Geometry: final body of the model. Coordinates: model frame, mm. A direction names the side the tool comes from. Give positions to 0.01 mm unless a question says otherwise; leave off trailing zeros. Write each loop counter-clockwise with the first axis right and the second up, starting at its lowest first coordinate (ties: lowest second). Pieces come first, ordered by that corner, then holes. Notation, with made-up numbers: M 62,38.5 L 109,38.5 A19 ccw 109,59.5 Z; hole C 32,85 d2. An arc over 180 degrees is marked long. Use a Markdown table: item, result. Add a question column.
(1) Reachability of faces 3 (the flat face through (2, -5, -32)), 4 (the flat face through (15.304, 32.045, -19.867)), 5 (the flat face through (-20, 32, -32.483)), 6 (the flat face through (-16, 1, -12.797)) from +Z, -Z, +X, -X, +Y, -Y: full face, straight path, thin tool, end or side. Return the list, or none.
(2) Cut plane B-B (x = 0). Output: boundary loops of the cut face in (y, z).
(3) Pin query (flat end, axial travel): pin 1 Ø1.2 at (x, y) = (-16, 2) entering from +Z; pin 2 Ø1.2 at (x, z) = (-16.5, -17.5) entering from -Y; pin 3 Ø2.5 at (x, y) = (-16, 1) entering from -Z; pin 4 Ø22.5 at (x, z) = (1, -36.5) entering from -Y. Return the tip coordinate at first contact, or that it passes through.
(4) Cut plane D-D (y = 27.5). Output: boundary loops of the cut face in (x, z), plus the area to 3 significant figures.
(5) Cut plane A-A (z = 0). Output: boundary loops of the cut face in (x, y).
(6) Cut plane C-C (y = 18). Output: boundary loops of the cut face in (x, z).
(7) Material intervals for L1, parallel to Z at x = 0, y = -4; L2, parallel to Y at x = -7.5, z = 0; L3, parallel to Y at x = -19.5, z = -21, sorted ascending.
(8) Draft query along Z for faces 1 (the cylindrical face through (7.63, -3.52, -37.56)), 2 (the flat face through (-5, 65, -20)). Return one class per face: released by +Z, released by -Z, zero draft, split by the parting line, or undercut.
Autodesk Inventor part; units mm, degrees
ref_plane "YZ Plane" through (0, 0, 0) normal (1, 0, 0) x (0, 1, 0)
ref_plane "XZ Plane" through (0, 0, 0) normal (0, 1, 0) x (-1, 0, 0)
ref_plane "XY Plane" through (0, 0, 0) normal (0, 0, 1) x (1, 0, 0)
sketch "Esquisse7" plane through (0, 0, 0) normal (0, 1, 0) x (-1, 0, 0)
  circle A0 centre (0, 0) radius 15
  circle A1 centre (0, -39.9666) radius 15
  line L0 (13, -7.4833) -> (-13, -7.4833)
  line L1 (-13, -7.4833) -> (-13, -32.4833)
  line L2 (-13, -32.4833) -> (13, -32.4833)
  line L3 (13, -32.4833) -> (13, -7.4833)
  dimension "d39" = 30
  dimension "d40" = 25
  dimension "d41" = 26
extrude "Extrusion7" add sketch "Esquisse7" along normal blind 65
sketch "Esquisse8" plane through (-13, 0, -32.4833) normal (-1, 0, 0) x (0, 0, 1)
  line L0 (0, 0) -> (25, 0) construction
  line L1 (25, 0) -> (25, 65) construction
  line L2 (0, 65) -> (25, 65) construction
  line L3 (0, 0) -> (0, 65) construction
  line L4 (25, 0) -> (0, 0)
  line L5 (0, 0) -> (0, 65)
  line L6 (0, 65) -> (25, 65)
  line L7 (25, 65) -> (25, 0)
  point P0 (32.4833, 0)
extrude "Extrusion8" add sketch "Esquisse8" along normal blind 12
sketch "Esquisse9" plane through (0, 0, 0) normal (0, -1, 0) x (1, 0, 0)
  arc A0 (-13, -32.4833) -> (13, -32.4833) centre (0, -39.9666) ccw construction
  line L0 (13, -7.4833) -> (13, -32.4833) construction
  arc A1 (13, -7.4833) -> (-13, -7.4833) centre (0, 0) ccw construction
  line L1 (-13, -7.4833) -> (-25, -7.4833) construction
  line L2 (-25, -32.4833) -> (-25, -7.4833) construction
  line L3 (-13, -32.4833) -> (-25, -32.4833) construction
  line L4 (-13, -7.4833) -> (-25, -7.4833) construction
  line L5 (-15, -7.4833) -> (-15, -32.4833) construction
  line L6 (-13, -32.4833) -> (-25, -32.4833) construction
  line L7 (-15, -12.7966) -> (-17.3067, -12.7966)
  line L8 (-17.3067, -12.7966) -> (-17.3067, -27.5847)
  line L9 (-17.3067, -27.5847) -> (-15, -27.5847)
  line L10 (-15, -27.5847) -> (-15, -12.7966)
  point P0 (-15, -29.9833)
  dimension "d47" = 10
extrude "Extrusion9" cut sketch "Esquisse9" against normal blind 3
sketch "Esquisse10" plane through (0, 0, 0) normal (0, -1, 0) x (1, 0, 0)
  arc A0 (-13, -32.4833) -> (13, -32.4833) centre (0, -39.9666) ccw construction
  line L0 (13, -7.4833) -> (13, -32.4833) construction
  arc A1 (13, -7.4833) -> (-13, -7.4833) centre (0, 0) ccw construction
  line L1 (-13, -7.4833) -> (-25, -7.4833) construction
  line L2 (-25, -32.4833) -> (-25, -7.4833) construction
  line L3 (-13, -32.4833) -> (-25, -32.4833) construction
  circle A2 centre (0, 0) radius 11.5
  circle A3 centre (0, -39.9666) radius 11.5
  arc A4 (-13, -32.4833) -> (13, -32.4833) centre (0, -39.9666) ccw
  dimension "d58" = 23
extrude "Extrusion10" add sketch "Esquisse10" along normal blind 5
sketch "Esquisse11" plane through (0, -5, 0) normal (0, -1, 0) x (1, 0, 0)
  circle A0 centre (0, -39.9666) radius 11.5 construction
  circle A1 centre (0, 0) radius 11.5 construction
  circle A2 centre (0, 0) radius 8
  circle A3 centre (0, -39.9666) radius 8
  dimension "d54" = 16
extrude "Extrusion11" cut sketch "Esquisse11" against normal blind 3
fillet "Congé6" radius 20 2 edges at (13, 32.5, -7.4833) (13, 32.5, -32.4833)
draft "Dépouille de face1" angle 4 pull direction (0, 1, 0) faces at (13, 21.6667, -17.2095) (13.057, 21.6667, -29.813) (13.2275, 21.6667, -8.6539) (-14.4854, 43.3333, -43.862) (-14.0102, 43.3333, -5.3586) fixed edges at (13, 65, -19.9833) (13.2878, 65, -31.6853) (13.2878, 65, -8.2813) (-1.3678, 65, -54.9041) (-1.3678, 65, 14.9375)
properties part number "head1"
Answer list:
| question | item | result |
|---|---|---|
| 1 | face 3 | +Z, -Z, +X, -X, -Y |
| 1 | face 4 | +X, +Y |
| 1 | face 5 | -X, +Y |
| 1 | face 6 | -Y |
| 2 | outline | M -5,-51.47 L 0,-51.47 L 0,-59.51 L 65,-54.97 L 65,15 L 0,19.55 L 0,11.5 L -5,11.5 L -5,8 L -2,8 L -2,-8 L -5,-8 L -5,-11.5 L 0,-11.5 L 0,-28.47 L -5,-28.47 L -5,-31.97 L -2,-31.97 L -2,-47.97 L -5,-47.97 Z |
| 3 | pin 1 | z = 11.81 |
| 3 | pin 2 | y = 3 |
| 3 | pin 3 | z = -52.69 |
| 3 | pin 4 | y = -5 |
| 4 | outline | M -25,-32.48 L -15.95,-32.48 A17.62 ccw long 16.62,-34.09 A17.38 cw 15.62,-28.3 L 15.62,-11.66 A17.38 cw 16.62,-5.87 A17.62 ccw long -15.95,-7.48 L -25,-7.48 Z |
| 4 | area | 2,500 mm² |
| 5 | outline | M -19.55,0 L -11.5,0 L -11.5,-5 L -8,-5 L -8,-2 L 8,-2 L 8,-5 L 11.5,-5 L 11.5,0 L 19.55,0 L 15,65 L -15,65 Z |
| 6 | outline | M -25,-32.48 L -16.69,-32.48 A18.29 ccw long 17.24,-33.87 A16.71 cw 16.29,-28.3 L 16.29,-11.66 A16.71 cw 17.24,-6.09 A18.29 ccw long -16.69,-7.48 L -25,-7.48 Z |
| 7 | L1 | -51.47 to -47.97, -31.97 to -28.47, -11.5 to -8, 8 to 11.5 |
| 7 | L2 | -2 to 65 |
| 7 | L3 | 0 to 65 |
| 8 | face 1 | undercut |
| 8 | face 2 | zero draft |
